```python
from build123d import *
from OCP.BRepFilletAPI import BRepFilletAPI_MakeChamfer

# Parameters (mm, degrees)
BOSS_EXTRUDE1_DEPTH = 15
CHAMFER1_SIZE       = 20
CHAMFER1_SIZE2      = 24.644345169
CHAMFER2_SIZE       = 20
CHAMFER2_SIZE2      = 24.644345169
CUT_EXTRUDE1_DEPTH  = 455.278391079
BOSS_EXTRUDE2_DEPTH = 15


with BuildPart() as part:
    # Sketch2 → Boss-Extrude1 (new body)
    with BuildSketch(Plane(origin=(0, 0, 0), x_dir=(1, 0, 0), z_dir=(0, 1, 0))):
        Polygon((-190.630365757, 0), (-225, -394.358791714), (-184.655281407, -394.358791714), (-126.173678801, -62.046246538), (126.173678801, -62.046246538), (184.655281407, -394.358791714), (225, -394.358791714), (190.630365757, 0), align=None)
    extrude(amount=-BOSS_EXTRUDE1_DEPTH)

    # Chamfer1: one chamfer whose edges measure the first distance from different faces: ONE call of the kernel's chamfer builder (chamfer() names one face for all edges)
    chamfer1_edges_1 = [part.edges().sort_by_distance(p)[0] for p in [
        (184.655281407, -7.5, 394.358791714),
    ]]
    chamfer1_side_1 = [part.faces().sort_by_distance(p)[0] for p in [
        (204.827640703, -7.5, 394.358791714),
    ]]
    chamfer1_edges_2 = [part.edges().sort_by_distance(p)[0] for p in [
        (-184.655281407, -7.5, 394.358791714),
    ]]
    chamfer1_side_2 = [part.faces().sort_by_distance(p)[0] for p in [
        (-204.827640703, -7.5, 394.358791714),
    ]]
    chamfer1 = BRepFilletAPI_MakeChamfer(part.part.solid().wrapped)
    for e in chamfer1_edges_1:
        chamfer1.Add(CHAMFER1_SIZE, CHAMFER1_SIZE2, e.wrapped, chamfer1_side_1[0].wrapped)  # the first distance lies on this face
    for e in chamfer1_edges_2:
        chamfer1.Add(CHAMFER1_SIZE, CHAMFER1_SIZE2, e.wrapped, chamfer1_side_2[0].wrapped)  # the first distance lies on this face
    add(Compound.cast(chamfer1.Shape()), mode=Mode.REPLACE)

    # Chamfer2: one chamfer whose edges measure the first distance from different faces: ONE call of the kernel's chamfer builder (chamfer() names one face for all edges)
    chamfer2_edges_1 = [part.edges().sort_by_distance(p)[0] for p in [
        (126.173678801, -7.5, 62.046246538),
    ]]
    chamfer2_side_1 = [part.faces().sort_by_distance(p)[0] for p in [
        (153.278797334, -7.5, 216.066836355),
    ]]
    chamfer2_edges_2 = [part.edges().sort_by_distance(p)[0] for p in [
        (-126.173678801, -7.5, 62.046246538),
    ]]
    chamfer2_side_2 = [part.faces().sort_by_distance(p)[0] for p in [
        (0, -7.5, 62.046246538),
    ]]
    chamfer2 = BRepFilletAPI_MakeChamfer(part.part.solid().wrapped)
    for e in chamfer2_edges_1:
        chamfer2.Add(CHAMFER2_SIZE, CHAMFER2_SIZE2, e.wrapped, chamfer2_side_1[0].wrapped)  # the first distance lies on this face
    for e in chamfer2_edges_2:
        chamfer2.Add(CHAMFER2_SIZE, CHAMFER2_SIZE2, e.wrapped, chamfer2_side_2[0].wrapped)  # the first distance lies on this face
    add(Compound.cast(chamfer2.Shape()), mode=Mode.REPLACE)

    # Sketch3 → Cut-Extrude1 (cut, through all)
    with BuildSketch(Plane(origin=(0, 0, 0), x_dir=(1, 0, 0), z_dir=(0, 1, 0))):
        Polygon((-196.037895257, -62.046246538), (-181.094105963, -63.348645731), (-175.573068194, 0), (-190.630365757, 0), align=None)
        Polygon((-210.518947628, -228.202519126), (-195.575158335, -229.504918319), (-200.402175792, -284.890342515), (-215.345965086, -283.587943322), align=None)
        Polygon((-220.172982543, -338.973367518), (-225, -394.358791714), (-209.942702437, -394.358791714), (-205.229193249, -340.275766711), align=None)
        Polygon((-200.864912714, -117.431670734), (-205.691930171, -172.81709493), (-190.748140877, -174.119494123), (-185.92112342, -118.734069927), align=None)
    cut_extrude1 = extrude(amount=-CUT_EXTRUDE1_DEPTH, mode=Mode.SUBTRACT)

    # Mirror1: Cut-Extrude1 across plane
    add(cut_extrude1.mirror(Plane(origin=(0, 0, 0), x_dir=(0, 0, 1), z_dir=(1, 0, 0))), mode=Mode.SUBTRACT)

    # Sketch5 → Boss-Extrude2 (add)
    with BuildSketch(Plane(origin=(0, 0, 0), x_dir=(1, 0, 0), z_dir=(0, 1, 0))):
        Polygon((-22.687908556, 0), (22.687908556, 0), (22.346610744, 13.033637599), (-22.346610744, 13.033637599), align=None)
    extrude(amount=-BOSS_EXTRUDE2_DEPTH)


solid = part.part
```
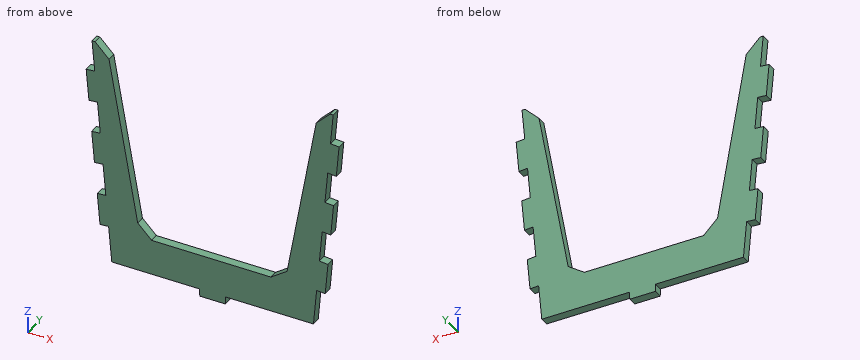
Here's how the part is built. I have some questions about the finished solid (model axes, mm). Round coordinates to 2 decimals unless told otherwise and drop trailing zeros. Loops run counter-clockwise (first coordinate to the right, second up) from the corner with the lowest first, then second, coordinate; pieces in that order, holes last. Notation, with made-up numbers: (-24, -9) -> (2, -9) arc R27 cw to (2, 8) -> close; hole circle Ø9 at (45, -19). An arc over 180 degrees is marked (long way). Answer as CSV lines item,"result".
1. If we section it at C-C on z = 206: Please give me the cut outline in (x, y).
Final values:
outline,"(-208.58, -15) -> (-151.51, -15) -> (-151.51, 0) -> (-208.58, 0) -> close; (151.51, -15) -> (208.58, -15) -> (208.58, 0) -> (151.51, 0) -> close"
2. If we section it at D-D on x = -44: Please give me the cut outline in (y, z), plus the area to 3 significant figures.
Final values:
outline,"(-15, 0) -> (0, 0) -> (0, 62.05) -> (-15, 62.05) -> close"
area,"931 mm^2"
3. If we section it at B-B on x = 17: Please give me the cut outline in (y, z), plus the area to 3 significant figures.
Final values:
outline,"(-15, -13.03) -> (0, -13.03) -> (0, 62.05) -> (-15, 62.05) -> close"
area,"1,130 mm^2"
4. For pin 1 (8 mm diameter, centred on x = -67.5, y = -6.5, fed in from -Z); pin 2 (4 mm diameter, centred on y = -9, z = 210.5, fed in from +X); pin 3 (2 mm diameter, centred on y = -10, z = 170, fed in from +X), each with a flat end and sliding along its axis, tell me the tip position at first contact or that it passes through.
Final values:
pin 1,"stops at z = 0"
pin 2,"stops at x = 209.15"
pin 3,"stops at x = 190.48"
5. If I drill on L1, parallel to Z at x = 6, y = -10.75; L2, parallel to X at y = -7, z = 277; L3, parallel to Z at x = -58, y = -9, over which ranges is the centre line in solid material (lowest first)?
Final values:
L1,"z = -13.03 to 62.05"
L2,"x = -199.71 to -164, 164 to 199.71"
L3,"z = 0 to 62.05"
6. If we section it at A-A on z = 74.5: Please give me the cut outline in (x, y).
Final values:
outline,"(-197.12, -15) -> (-118.63, -15) -> (-118.63, 0) -> (-197.12, 0) -> close; (119.3, -15) -> (197.12, -15) -> (197.12, 0) -> (119.3, 0) -> close"
